Could you check a few things on this model? Use its own coordinates, in mm. Give positions to 0.01 mm unless a question says otherwise; leave off trailing zeros. Write each loop counter-clockwise with the first axis right and the second up, starting at its lowest first coordinate (ties: lowest second). Pieces come first, ordered by that corner, then holes. Notation, with made-up numbers: M 48.25,79.25 L 103.25,79.25 A17 ccw 103.25,99.25 Z; hole C 49,52.5 d4. An arc over 180 degrees is marked long. Answer as CSV lines item,"result". Start each with the question number.
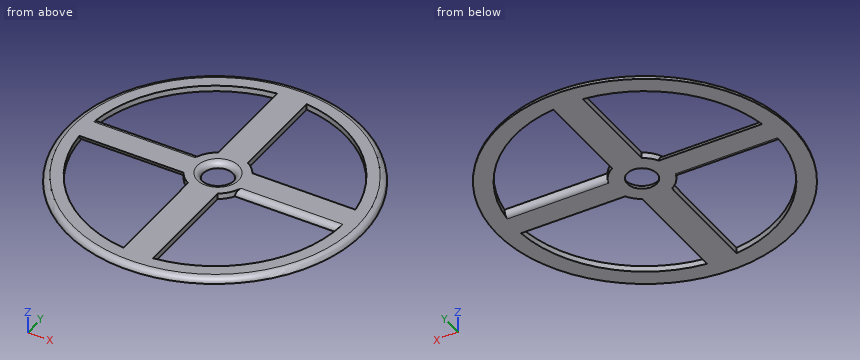
from build123d import *

# Parameters (mm, degrees)
F0_R     = 50
F0_R_2   = 5
F1_DEPTH = 2
F2_R     = 1.99999


# Not quite as in the source:
# - a fillet or chamfer is up to 0.001 mm smaller than in the source, because OpenCascade refuses the exact size


with BuildPart() as f1:
    # F0 (on Top) → F1 (new body)
    with BuildSketch(Plane.XY):
        with Locations((0, -1.6630436294)):
            Circle(F0_R)
        with BuildLine():
            ThreePointArc((-5, -45.3780296182), (-31.6977238962, -32.1795031194), (-43.873280276, -5))
            Line((-43.873280276, -5), (-8.6602540378, -5))
            ThreePointArc((-8.6602540378, -5), (-7.0710678119, -7.0710678119), (-5, -8.6602540378))
            Line((-5, -8.6602540378), (-5, -45.3780296182))
        make_face(mode=Mode.SUBTRACT)
        with BuildLine():
            ThreePointArc((5, -8.6602540378), (7.0710678119, -7.0710678119), (8.6602540378, -5))
            Line((8.6602540378, -5), (43.873280276, -5))
            ThreePointArc((43.873280276, -5), (31.6977238962, -32.1795031194), (5, -45.3780296182))
            Line((5, -45.3780296182), (5, -8.6602540378))
        make_face(mode=Mode.SUBTRACT)
        with BuildLine():
            ThreePointArc((-43.4925723497, 5), (-30.513832952, 30.0372087131), (-5, 42.0519423594))
            Line((-5, 42.0519423594), (-5, 8.6602540378))
            ThreePointArc((-5, 8.6602540378), (-7.0710678119, 7.0710678119), (-8.6602540378, 5))
            Line((-8.6602540378, 5), (-43.4925723497, 5))
        make_face(mode=Mode.SUBTRACT)
        Circle(F0_R_2, mode=Mode.SUBTRACT)
        with BuildLine():
            Line((43.4925723497, 5), (8.6602540378, 5))
            ThreePointArc((8.6602540378, 5), (7.0710678119, 7.0710678119), (5, 8.6602540378))
            Line((5, 8.6602540378), (5, 42.0519423594))
            ThreePointArc((5, 42.0519423594), (30.513832952, 30.0372087131), (43.4925723497, 5))
        make_face(mode=Mode.SUBTRACT)
    extrude(amount=F1_DEPTH)

    # F2 (radius 2 in the source; OpenCascade refuses exactly that, so slightly less here)
    f2_edges = [f1.edges().sort_by_distance(p)[0] for p in [
        (-50, -1.663044, 2),
        (26.076413, 5, 0),
        (-26.266767, -5, 0),
        (-26.076413, 5, 2),
        (26.266767, -5, 2),
        (-5, 0, 2),
    ]]
    fillet(f2_edges, radius=F2_R)


solid = f1.part
1. Imagine slicing it at C-C, the plane y = 37.5. State how many separate pieces and enclosed holes the cut face has, plus the area to 3 significant figures.
2. Please list where these lines run through material, in increasing order: line 1 (X direction, y = -37, z = 1.6); line 2 (X direction, y = -9, z = 1.1); line 3 (Y direction, x = 30.5, z = 1.25).
3. Imagine slicing it at B-B, the plane z = 0.95. Please give me the cut outline in (x, y), plus the area to 3 significant figures.
4. Will these pins go through, and if not, where does the flat tip stop? P1, Ø1, axis at y = -19, z = 0, coming from the +X side; P2, Ø0.6, axis at y = -34, z = 1, coming from the +X side; P3, Ø16, axis at x = 0, y = 0, coming from the -Z side; P4, Ø1, axis at x = -20, z = 1.5, coming from the -Y side.
Solutions:
1,separate pieces,"3"
1,enclosed holes,"0"
1,area,"61.3 mm²"
2,line 1,"-34.23 to -26.22, -5 to 5, 26.22 to 34.23"
2,line 2,"-49.13 to -43.38, -5 to 5, 43.38 to 49.13"
2,line 3,"-40.73 to -33.38, -4.56 to 4.85, 30.05 to 37.4"
3,outline,"C 0,-1.66 d99.52; hole M -43.89,-4.7 A44 ccw -5,-45.38 L -5,-8.66 A10 cw -8.83,-4.7 Z; hole M -43.53,4.76 L -8.79,4.76 A10 cw -5,8.66 L -5,42.05 A44 ccw Z; hole C 0,0 d10.48; hole M 5,-45.38 A44 ccw 43.89,-4.76 L 8.79,-4.76 A10 cw 5,-8.66 Z; hole M 5,8.66 A10 cw 8.83,4.7 L 43.54,4.7 A44 ccw 5,42.05 Z"
3,area,"3,260 mm²"
4,P1,"x = 47.08"
4,P2,"x = 38.11"
4,P3,"z = 0"
4,P4,"y = -47.26"
